from build123d import *

# Parameters (mm, degrees)
EXTRUDE_1_DEPTH          = 6.86
SKETCH_3_R               = 14
EXTRUDE_2_DEPTH          = 140
SKETCH_4_R               = 14
EXTRUDE_3_DEPTH          = 9.54
EXTRUDE_START            = 8.87
SKETCH_5_R               = 14
EXTRUDE_4_DEPTH          = 8.87
SKETCH_6_W               = 40
SKETCH_6_H               = 51.5
EXTRUDE_5_DEPTH          = 50
CUT_EXTRUDE_1_DEPTH      = 70
SKETCH_8_W               = 58.379913489
SKETCH_8_H               = 45.5
CUT_EXTRUDE_2_DEPTH      = 50
SKETCH_9_R               = 5
CUT_EXTRUDE_3_DEPTH      = 60
EXTRUDE_6_DEPTH          = 6.86
SKETCH_11_R              = 6
CUT_EXTRUDE_4_DEPTH      = 6.86
CUT_EXTRUDE_5_DEPTH      = 218.354242016
CUT_EXTRUDE_5_DEPTH_BACK = 218.354242016
SKETCH_12_R              = 5
CUT_EXTRUDE_6_DEPTH      = 6.86
CUT_EXTRUDE_7_DEPTH      = 6.86
FILLET_1_R               = 10
FILLET_2_R               = 10


with BuildPart() as part:
    # 스케치1 → 보스-돌출1 (new body)
    with BuildSketch(Plane.XY):
        Polygon((-140.292347602, 27.740456746), (-140.292347602, -32.259543254), (51.707652398, -62.259543254), (101.707652398, -62.259543254), (101.707652398, 77.740456746), (51.707652398, 77.740456746), align=None)
    extrude(amount=EXTRUDE_1_DEPTH)

    # 스케치3 → 보스-돌출2 (add)
    with BuildSketch(Plane(origin=(0, 77.740456746, 0), x_dir=(1, 0, 0), z_dir=(0, 1, 0))):
        with Locations((87.707652398, -3.43)):
            Circle(SKETCH_3_R)
    extrude(amount=-EXTRUDE_2_DEPTH)

    # 스케치4 → 보스-돌출3 (add)
    with BuildSketch(Plane.XZ.offset(62.259543254)):
        with Locations((87.707652398, 3.43)):
            Circle(SKETCH_4_R)
    extrude(amount=EXTRUDE_3_DEPTH)

    # 스케치5 → 보스-돌출4 (add)
    with BuildSketch(Plane(origin=(0, 77.740456746, 0), x_dir=(1, 0, 0), z_dir=(0, 1, 0)).offset(EXTRUDE_START)):
        with Locations(Location((87.707652398, -3.43, 0), (0, 0, 270))):
            Circle(SKETCH_5_R)
    extrude(amount=-EXTRUDE_4_DEPTH)

    # 스케치6 → 보스-돌출5 (add)
    with BuildSketch(Plane(origin=(0, 0, 0), x_dir=(-1, 0, 0), z_dir=(0, 0, -1))):
        with Locations((37.365670703, -59.549543254)):
            Rectangle(SKETCH_6_W, SKETCH_6_H)
    extrude(amount=EXTRUDE_5_DEPTH)

    # 스케치7 → 컷-돌출1 (cut)
    with BuildSketch(Plane.XZ.offset(85.299543254)):
        with BuildLine():
            Line((-57.365670703, -31.410504054), (-57.365670703, -50))
            Line((-57.365670703, -50), (-17.365670703, -50))
            Line((-17.365670703, -50), (-17.365670703, -31.410504054))
            ThreePointArc((-17.365670703, -31.410504054), (-37.365670703, -49.67087302), (-57.365670703, -31.410504054))
        make_face()
    extrude(amount=-CUT_EXTRUDE_1_DEPTH, mode=Mode.SUBTRACT)

    # 스케치8 → 컷-돌출2 (cut)
    with BuildSketch(Plane(origin=(-17.365670703, 0, 0), x_dir=(0, 0, -1), z_dir=(1, 0, 0))):
        with Locations((32.189956745, -59.549543254)):
            Rectangle(SKETCH_8_W, SKETCH_8_H)
    extrude(amount=-CUT_EXTRUDE_2_DEPTH, mode=Mode.SUBTRACT)

    # 스케치9 → 컷-돌출3 (cut)
    with BuildSketch(Plane.XZ.offset(85.299543254)):
        with Locations((-37.365670703, -29.58800733)):
            Circle(SKETCH_9_R)
    extrude(amount=-CUT_EXTRUDE_3_DEPTH, mode=Mode.SUBTRACT)

    # 스케치10 → 보스-돌출6 (add)
    with BuildSketch(Plane.XY):
        Polygon((-17.365670703, -51.466836519), (-17.365670703, -85.299543254), (-57.365670703, -85.299543254), (-57.365670703, -45.216836519), align=None)
    extrude(amount=EXTRUDE_6_DEPTH)

    # 스케치11 → 컷-돌출4 (cut)
    with BuildSketch(Plane(origin=(0, 0, 0), x_dir=(-1, 0, 0), z_dir=(0, 0, -1))):
        with Locations((100.292347602, -2.259543254)):
            Circle(SKETCH_11_R)
        with Locations((125.292347602, -2.259543254)):
            Circle(SKETCH_11_R)
    extrude(amount=-CUT_EXTRUDE_4_DEPTH, mode=Mode.SUBTRACT)

    # 스케치12 → 컷-돌출5 (cut, two sides: drawn at the far end of the back side and taken through both)
    with BuildSketch(Plane.XZ.offset(71.799543254).offset(-CUT_EXTRUDE_5_DEPTH_BACK)):
        with Locations((87.707652398, 3.43)):
            Circle(SKETCH_12_R)
    extrude(amount=CUT_EXTRUDE_5_DEPTH + CUT_EXTRUDE_5_DEPTH_BACK, mode=Mode.SUBTRACT)

    # 스케치13 → 컷-돌출6 (cut)
    with BuildSketch(Plane(origin=(0, 0, 0), x_dir=(-1, 0, 0), z_dir=(0, 0, -1))):
        Polygon((-74.134329297, 50.339076342), (-30.453327594, 50.339076342), (0, 43.027707352), (0, -29.365200476), (-30.453327594, -36.922211026), (-74.134329297, -36.922211026), align=None)
    extrude(amount=-CUT_EXTRUDE_6_DEPTH, mode=Mode.SUBTRACT)

    # 스케치14 → 컷-돌출7 (cut)
    with BuildSketch(Plane(origin=(0, 0, 0), x_dir=(-1, 0, 0), z_dir=(0, 0, -1))):
        Polygon((68.524633072, 24.49831751), (36.848219376, 30.426812619), (36.848219376, -24.572302869), (68.524633072, -17.60850751), align=None)
    extrude(amount=-CUT_EXTRUDE_7_DEPTH, mode=Mode.SUBTRACT)

    # 필렛1
    fillet_1_edges = [part.edges().sort_by_distance(p)[0] for p in [
        (0, 43.027707352, 3.43),
        (0, -29.365200476, 3.43),
        (-68.524633072, 24.49831751, 3.43),
        (-68.524633072, -17.60850751, 3.43),
        (-36.848219376, -24.572302869, 3.43),
        (-36.848219376, 30.426812619, 3.43),
    ]]
    fillet(fillet_1_edges, radius=FILLET_1_R)

    # 필렛2
    fillet_2_edges = [part.edges().sort_by_distance(p)[0] for p in [
        (-140.292347602, -32.259543254, 3.43),
        (-140.292347602, 27.740456746, 3.43),
    ]]
    fillet(fillet_2_edges, radius=FILLET_2_R)


solid = part.part
Input: part model. Units: mm. Frame: model coordinates. A direction names the side the tool comes from. Give positions to 0.01 mm unless a question says otherwise; leave off trailing zeros. Write each loop counter-clockwise with the first axis right and the second up, starting at its lowest first coordinate (ties: lowest second). Pieces come first, ordered by that corner, then holes. Notation, with made-up numbers: M 50,-21 L 103,-21 A25 ccw 103,2 Z; hole C 89,49.5 d9. An arc over 180 degrees is marked long. Write item = value, one per line. Start each with the question number.
1) Material intervals for line 1 along Y through (x, z) = (-42.5, -42.5); line 2 along Z through (x, y) = (-113, -23); line 3 along Y through (x, z) = (48, 3), sorted ascending. Write a range as [from, to].
2) Draft query along Y for faces 1 (the flat face through (-140.292, -2, 3)), 2 (the flat face through (-95.122, -39.317, 3.382)), 3 (the flat face through (-37, -82.3, -21)). Return one class per face: +Y half, -Y half, draft (parallel to the pull), parting line (faces both ways), or undercut.
3) Cut plane B-B on y = 61. Return the cut outline in (x, z), then the cut area to 3 significant figures.
4) Cut plane A-A on z = -40.5. Return the cut outline in (x, y), then the cut area to 3 significant figures.
5) Reachability of faces 4 (the flat face through (101.708, 7, 3)), 5 (the flat face through (74.134, 6, 3)), 6 (the flat face through (-17.366, -63, -1)) from +Z, -Z, +X, -X, +Y, -Y: full face, straight path, thin tool, end or side. Return the list, or none.
6) First-contact query: pin 1 Ø14 at (x, y) = (-125.29, -2.26) entering from +Z; pin 2 Ø13 at (x, z) = (87.71, 3.43) entering from -Y; pin 3 Ø5.5 at (x, z) = (60.5, 2) entering from -Y. Flat tips, straight axial feed; report the tip coordinate or a pass-through.
Solved:
q1.line_1 = [-85.3, -82.3], [-36.8, -33.8]
q1.line_2 = [0, 6.86]
q1.line_3 = [-61.68, -36.92], [50.34, 76.77]
q2.face_1 = draft
q2.face_2 = -Y half
q2.face_3 = undercut
q3.outline = M -12.58,0 L 74.13,0 A14 ccw 101.28,0 L 101.71,0 L 101.71,6.86 L 101.28,6.86 A14 ccw 74.13,6.86 L -12.58,6.86 Z; hole C 87.71,3.43 d10
q3.area = 1,130 mm2
q4.outline = M -54.23,-85.3 L -20.51,-85.3 L -20.51,-82.3 L -54.23,-82.3 Z; M -54.23,-36.8 L -20.51,-36.8 L -20.51,-33.8 L -54.23,-33.8 Z
q4.area = 202 mm2
q5.face_4 = +Z, -Z, +X, +Y, -Y
q5.face_5 = +Z, -Z
q5.face_6 = -Z, -Y
q6.pin_1 = 6.86
q6.pin_2 = -71.8
q6.pin_3 = -62.26
